from build123d import *

# Parameters (mm, degrees)
SKETCH1_W           = 40
SKETCH1_H           = 40
BOSS_EXTRUDE1_DEPTH = 40
SKETCH2_W           = 20
SKETCH2_H           = 20
CUT_EXTRUDE1_DEPTH  = 40
SKETCH3_W           = 20
SKETCH3_H           = 20
CUT_EXTRUDE2_DEPTH  = 40
CUT_EXTRUDE3_DEPTH  = 20


with BuildPart() as part:
    # Sketch1 → Boss-Extrude1 (new body)
    with BuildSketch(Plane.XY):
        with Locations((20, 20)):
            Rectangle(SKETCH1_W, SKETCH1_H)
    extrude(amount=BOSS_EXTRUDE1_DEPTH)

    # Sketch2 → Cut-Extrude1 (cut)
    with BuildSketch(Plane.XY.offset(40)):
        with Locations((10, 30)):
            Rectangle(SKETCH2_W, SKETCH2_H)
    extrude(amount=-CUT_EXTRUDE1_DEPTH, mode=Mode.SUBTRACT)

    # Sketch3 → Cut-Extrude2 (cut)
    with BuildSketch(Plane.ZY.offset(-20)):
        with Locations((30, 30)):
            Rectangle(SKETCH3_W, SKETCH3_H)
    extrude(amount=-CUT_EXTRUDE2_DEPTH, mode=Mode.SUBTRACT)

    # Sketch4 → Cut-Extrude3 (cut)
    with BuildSketch(Plane.XY.offset(40)):
        Polygon((0, 20), (20, 0), (0, 0), align=None)
    extrude(amount=-CUT_EXTRUDE3_DEPTH, mode=Mode.SUBTRACT)


solid = part.part
Model file for the job. Use its own axes, mm. A direction names the side the tool comes from. Coordinates: 2 decimals unless noted, no trailing zeros. Write each loop counter-clockwise with the first axis right and the second up, starting at its lowest first coordinate (ties: lowest second). Pieces come first, ordered by that corner, then holes. Notation, with made-up numbers: (-8.75, 34.5) -> (18.25, 34.5) arc R33 cw to (18.25, 71.5) -> close; hole circle Ø3 at (63.25, 89). An arc over 180 degrees is marked (long way). One line per item, written item: value. Start each with the question number.
1) Flat gauge pins, fed straight in: pin 1 Ø10 at (y, z) = (26, 14.5) entering from -X; pin 2 Ø3 at (y, z) = (19.5, 35.5) entering from -X. Where does each tip first touch, or does it go through?
2) Which spindle directions (+Z, -Z, +X, -X, +Y, -Y) get a long thin tool onto all of the face, cutting with end or side? Do faces 1 (the face through (20, 30, 10)), 2 (the face through (24, 16, 0)), 3 (the face through (10, 10, 30)), 4 (the face through (24, 0, 15)), 5 (the face through (30, 30, 20)). Say none if no direction does.
3) Slice it at A-A on y = 3. Write the cut outline in (x, z), then the cut area to 3 significant figures.
4) Slice it at B-B on x = 8. Write the cut outline in (y, z), then the cut area to 3 significant figures.
5) Slice it at D-D on y = 29. Write the cut outline in (x, z), then the cut area to 3 significant figures.
6) Probe probe 1 along Z at (x, y) = (32.5, 35); probe 2 along X at (y, z) = (28, 16.5). List the from-to ranges inside material, lowest first.
7) Slice it at C-C on z = 23.5. Write the cut outline in (x, y).
Answers follow:
1. pin 1: x = 20
1. pin 2: x = 0
2. face 1: +Z, -Z, -X, +Y
2. face 2: -Z, +X, -X, +Y, -Y
2. face 3: +Z, -X, -Y
2. face 4: +Z, -Z, +X, -X, -Y
2. face 5: +Z, +X, -X, +Y
3. outline: (0, 0) -> (40, 0) -> (40, 40) -> (17, 40) -> (17, 20) -> (0, 20) -> close
3. area: 1,260 mm2
4. outline: (0, 0) -> (20, 0) -> (20, 40) -> (12, 40) -> (12, 20) -> (0, 20) -> close
4. area: 560 mm2
5. outline: (20, 0) -> (40, 0) -> (40, 20) -> (20, 20) -> close
5. area: 400 mm2
6. probe 1: 0 to 20
6. probe 2: 20 to 40
7. outline: (0, 20) -> (20, 0) -> (40, 0) -> (40, 20) -> close
